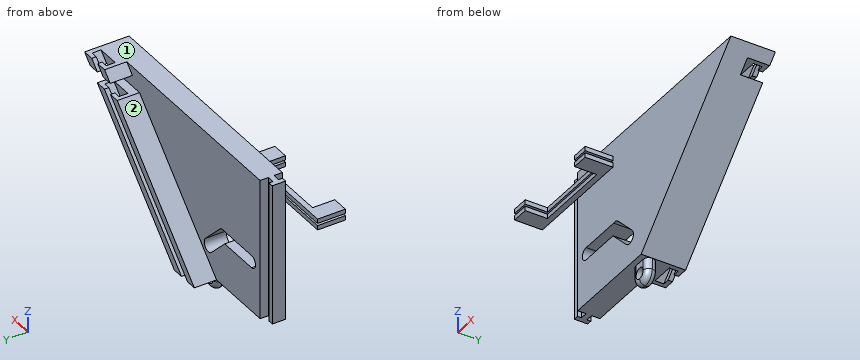
```python
from build123d import *

# Parameters (mm, degrees)
BOSS_EXTRUDE1_DEPTH  = 10
BOSS_EXTRUDE3_DEPTH  = 65
SKETCH3_W            = 6.566984135
SKETCH3_H            = 1.360389693
CUT_EXTRUDE2_DEPTH   = 65
BOSS_EXTRUDE4_DEPTH  = 3.25
BOSS_EXTRUDE5_DEPTH  = 2.25
SKETCH7_W            = 10
SKETCH7_H            = 5
BOSS_EXTRUDE6_DEPTH  = 10
SKETCH8_R            = 2.5
CUT_EXTRUDE3_DEPTH   = 10
FILLET1_R            = 5
FILLET2_R            = 5
FILLET4_R            = 2.5
FILLET5_R            = 2.5
SKETCH9_W            = 100
SKETCH9_H            = 5.5
CUT_EXTRUDE4_DEPTH   = 100
BOSS_EXTRUDE7_DEPTH  = 10
CUT_EXTRUDE5_DEPTH   = 150
SKETCH12_W           = 29.92089387
SKETCH12_H           = 33.203721342
CUT_EXTRUDE6_DEPTH   = 150
SKETCH14_W           = 19.184954217
SKETCH14_H           = 28.132637814
CUT_EXTRUDE7_DEPTH   = 150
SKETCH16_W           = 15.620456736
SKETCH16_H           = 10.822807293
CUT_EXTRUDE8_DEPTH   = 150
CUT_EXTRUDE9_DEPTH   = 10
CUT_EXTRUDE10_DEPTH  = 10
SKETCH19_W           = 10
SKETCH19_H           = 2
SKETCH19_W_2         = 15
BOSS_EXTRUDE9_DEPTH  = 2.5
SKETCH21_W           = 7.5
SKETCH21_H           = 2
BOSS_EXTRUDE10_DEPTH = 10


with BuildPart() as part:
    # Sketch1 → Boss-Extrude1 (new body)
    with BuildSketch(Plane(origin=(0, 0, 0), x_dir=(1, 0, 0), z_dir=(0, 1, 0))):
        Polygon((-11.672910159, -34.563988547), (96.966700148, -34.563988547), (33.327089841, 29.07562176), (-11.672910159, 29.07562176), align=None)
    extrude(amount=BOSS_EXTRUDE1_DEPTH)

    # Sketch2 → Boss-Extrude3 (add)
    with BuildSketch(Plane.XY.offset(34.563988547)):
        Polygon((-11.672910159, 3.75), (-14.922910159, 3.75), (-14.922910159, 2), (-17.172910159, 2), (-17.172910159, 8), (-14.922910159, 8), (-14.922910159, 6.25), (-11.672910159, 6.25), align=None)
    extrude(amount=-BOSS_EXTRUDE3_DEPTH)

    # Sketch3 → Cut-Extrude2 (cut)
    with BuildSketch(Plane(origin=(0, 8, 0), x_dir=(1, 0, 0), z_dir=(0, 1, 0))):
        with Locations((-13.889418092, 29.755816607)):
            Rectangle(SKETCH3_W, SKETCH3_H)
    extrude(amount=-CUT_EXTRUDE2_DEPTH, mode=Mode.SUBTRACT)

    # Sketch4 → Boss-Extrude4 (add)
    with BuildSketch(Plane(origin=(0, 10, 0), x_dir=(1, 0, 0), z_dir=(0, 1, 0))):
        Polygon((91.663399289, -34.563988547), (28.023788982, 29.07562176), (25.520630977, 29.07562176), (89.160241283, -34.563988547), align=None)
    extrude(amount=BOSS_EXTRUDE4_DEPTH)

    # Sketch6 → Boss-Extrude5 (add)
    with BuildSketch(Plane(origin=(0, 13.25, 0), x_dir=(1, 0, 0), z_dir=(0, 1, 0))):
        Polygon((90.411820286, -34.563988547), (94.136820286, -34.563988547), (30.497209979, 29.07562176), (23.047209979, 29.07562176), (86.686820286, -34.563988547), align=None)
    extrude(amount=BOSS_EXTRUDE5_DEPTH)

    # Sketch7 → Boss-Extrude6 (add)
    with BuildSketch(Plane(origin=(0, 0, -29.07562176), x_dir=(-1, 0, 0), z_dir=(0, 0, -1))):
        with Locations((-28.327089841, 5)):
            Rectangle(SKETCH7_W, SKETCH7_H)
    extrude(amount=BOSS_EXTRUDE6_DEPTH)

    # Sketch8 → Cut-Extrude3 (cut)
    with BuildSketch(Plane(origin=(0, 7.5, 0), x_dir=(1, 0, 0), z_dir=(0, 1, 0))):
        with Locations(Location((28.327089841, 34.07562176, 0), (0, 0, 270))):
            Circle(SKETCH8_R)
    extrude(amount=-CUT_EXTRUDE3_DEPTH, mode=Mode.SUBTRACT)

    # Fillet1
    fillet1_edges = [part.edges().sort_by_distance(p)[0] for p in [
        (23.327089841, 5, -39.07562176),
    ]]
    fillet(fillet1_edges, radius=FILLET1_R)

    # Fillet2
    fillet2_edges = [part.edges().sort_by_distance(p)[0] for p in [
        (33.327089841, 5, -39.07562176),
    ]]
    fillet(fillet2_edges, radius=FILLET2_R - 0.0001)  # a hair under: the kernel refuses the full size

    # Fillet4
    fillet4_edges = [part.edges().sort_by_distance(p)[0] for p in [
        (23.327089841, 7.5, -31.57562176),
        (33.327089841, 7.5, -31.57567176),
        (24.791555935, 7.5, -37.611155666),
    ]]
    fillet(fillet4_edges, radius=FILLET4_R - 0.0001)  # a hair under: the kernel refuses the full size

    # Fillet5
    fillet5_edges = [part.edges().sort_by_distance(p)[0] for p in [
        (23.327089841, 2.5, -31.57562176),
        (33.327089841, 2.5, -31.57567176),
        (24.791555935, 2.5, -37.611155666),
        (31.862653036, 2.5, -37.611184955),
    ]]
    fillet(fillet5_edges, radius=FILLET5_R - 0.0001)  # a hair under: the kernel refuses the full size

    # Sketch9 → Cut-Extrude4 (cut)
    with BuildSketch(Plane.XY.offset(34.563988547)):
        with Locations((44.136820286, 12.75)):
            Rectangle(SKETCH9_W, SKETCH9_H)
    extrude(amount=-CUT_EXTRUDE4_DEPTH, mode=Mode.SUBTRACT)

    # Sketch10 → Boss-Extrude7 (add)
    with BuildSketch(Plane(origin=(0, 10, 0), x_dir=(1, 0, 0), z_dir=(0, 1, 0))):
        Polygon((96.966700148, -34.563988547), (89.895632336, -41.635056358), (7.416994707, 40.84358127), (14.488062519, 47.914649082), align=None)
    extrude(amount=BOSS_EXTRUDE7_DEPTH)

    # Sketch11 → Cut-Extrude5 (cut)
    with BuildSketch(Plane(origin=(65.765344347, 0, 65.765344347), x_dir=(0.7071067811865475, 0, -0.7071067811865477), z_dir=(0.7071067811865477, 0, 0.7071067811865475))):
        Polygon((40.542543722, 20), (40.542543722, 18), (42.592543722, 18), (42.592543722, 14), (35.492543722, 14), (35.492543722, 18), (37.542543722, 18), (37.542543722, 20), align=None)
    extrude(amount=-CUT_EXTRUDE5_DEPTH, mode=Mode.SUBTRACT)

    # Sketch12 → Cut-Extrude6 (cut)
    with BuildSketch(Plane(origin=(0, 10, 0), x_dir=(-1, 0, 0), z_dir=(0, -1, 0))):
        with Locations((-34.145401152, 45.677482431)):
            Rectangle(SKETCH12_W, SKETCH12_H)
    extrude(amount=-CUT_EXTRUDE6_DEPTH, mode=Mode.SUBTRACT)


with BuildPart() as cut_extrude6_piece_1:
    # of the separate pieces the step leaves, piece 1, a body of its own (cut_extrude6_pieces)
    add(part.part.solids().sort_by_distance((30.827189841, 2.5, -29.07562176))[0])

    # Sketch16 → Cut-Extrude8 (cut)
    with BuildSketch(Plane(origin=(0, 10, 0), x_dir=(-1, 0, 0), z_dir=(0, -1, 0))):
        with Locations((-90.634792892, -39.975392193)):
            Rectangle(SKETCH16_W, SKETCH16_H)
    extrude(amount=-CUT_EXTRUDE8_DEPTH, mode=Mode.SUBTRACT)

    # Sketch17 → Cut-Extrude9 (cut)
    with BuildSketch(Plane(origin=(0, 20, 0), x_dir=(1, 0, 0), z_dir=(0, 1, 0))):
        Polygon((92.966700148, -30.563988547), (78.824564524, -30.563988547), (73.824564524, -25.563988547), (87.966700148, -25.563988547), align=None)
    extrude(amount=-CUT_EXTRUDE9_DEPTH, mode=Mode.SUBTRACT)

    # Sketch18 → Cut-Extrude10 (cut)
    with BuildSketch(Plane(origin=(0, 10, 0), x_dir=(1, 0, 0), z_dir=(0, 1, 0))):
        with BuildLine():
            Line((27.059004739, 14.493613639), (16.811162643, 4.245771544))
            ThreePointArc((16.811162643, 4.245771544), (12.674223335, 4.245771544), (12.674223335, 8.382710852))
            Line((12.674223335, 8.382710852), (22.92206543, 18.630552948))
            ThreePointArc((22.92206543, 18.630552948), (27.059004739, 18.630552948), (27.059004739, 14.493613639))
        make_face()
        with BuildLine():
            Line((14.742692989, 3.517272066), (-5.595455146, 3.517272066))
            ThreePointArc((-5.595455146, 3.517272066), (-8.392424278, 6.314241198), (-5.595455146, 9.11121033))
            Line((-5.595455146, 9.11121033), (14.742692989, 9.11121033))
            ThreePointArc((14.742692989, 9.11121033), (17.539662121, 6.314241198), (14.742692989, 3.517272066))
        make_face()
    extrude(amount=-CUT_EXTRUDE10_DEPTH, mode=Mode.SUBTRACT)

    # Sketch19 → Boss-Extrude9 (add)
    with BuildSketch(Plane(origin=(0, 0, 0), x_dir=(-1, 0, 0), z_dir=(0, -1, 0))):
        with Locations((-8.327089841, -26.563988547)):
            Rectangle(SKETCH19_W, SKETCH19_H)
        with Locations((-8.327089841, -23.563988547)):
            Rectangle(SKETCH19_W, SKETCH19_H)
        with Locations((31.672910159, -26.563988547)):
            Rectangle(SKETCH19_W, SKETCH19_H)
        with Locations((31.672910159, -23.563988547)):
            Rectangle(SKETCH19_W, SKETCH19_H)
        with Locations((4.172910159, -26.563988547)):
            Rectangle(SKETCH19_W_2, SKETCH19_H)
        with Locations((4.172910159, -23.563988547)):
            Rectangle(SKETCH19_W_2, SKETCH19_H)
        with Locations((19.172910159, -26.563988547)):
            Rectangle(SKETCH19_W_2, SKETCH19_H)
        with Locations((19.172910159, -23.563988547)):
            Rectangle(SKETCH19_W_2, SKETCH19_H)
    extrude(amount=BOSS_EXTRUDE9_DEPTH)

    # Sketch21 → Boss-Extrude10 (add)
    with BuildSketch(Plane(origin=(0, -2.5, 0), x_dir=(-1, 0, 0), z_dir=(0, -1, 0))):
        with Locations((-9.577089841, -23.563988547)):
            Rectangle(SKETCH21_W, SKETCH21_H)
        with Locations((-9.577089841, -26.563988547)):
            Rectangle(SKETCH21_W, SKETCH21_H)
        with Locations((32.922910159, -26.563988547)):
            Rectangle(SKETCH21_W, SKETCH21_H)
        with Locations((32.922910159, -23.563988547)):
            Rectangle(SKETCH21_W, SKETCH21_H)
    extrude(amount=BOSS_EXTRUDE10_DEPTH)


with BuildPart() as cut_extrude6_piece_2:
    # of the separate pieces the step leaves, piece 2, a body of its own (cut_extrude6_pieces)
    add(part.part.solids().sort_by_distance((7.416994707, 10, -40.84358127))[0])

    # Sketch14 → Cut-Extrude7 (cut)
    with BuildSketch(Plane(origin=(0, 10, 0), x_dir=(-1, 0, 0), z_dir=(0, -1, 0))):
        with Locations((-9.592477109, 43.141940667)):
            Rectangle(SKETCH14_W, SKETCH14_H)
    extrude(amount=-CUT_EXTRUDE7_DEPTH, mode=Mode.SUBTRACT)


solid = cut_extrude6_piece_1.part
```
CAD build for the part. Positions are in the model's coordinates, mm. Face numbers are marked on the shaded views. A direction names the side the tool comes from. Round coordinates to 2 decimals unless told otherwise and drop trailing zeros. Order: outer loops, then holes, each group sorted by start corner. A loop starts at its lowest first (then second) coordinate and runs counter-clockwise, first axis right, second up. Notation, with made-up numbers: (11.5, -5.75) -> (69.5, -5.75) arc R21 cw to (69.5, 22.25) -> close; hole circle Ø3 at (82.5, 71.5). An arc over 180 degrees is marked (long way). Write item = value, one per line.
(1) Flat gauge pins, fed straight in: P1, Ø0.6, axis at x = -17.5, z = 23.5, coming from the -Y side; P2, Ø1.9, axis at y = 2, z = -8.5, coming from the -X side; P3, Ø12, axis at x = -10, z = -31.5, coming from the +Y side. Where does each tip first touch, or does it go through?
Answers follow:
P1 = -2.5
P2 = -17.17
P3 = 10
(2) Cut at D-D (z = 2). Write the cut outline in (x, y).
Answers follow:
outline = (-17.17, 2) -> (-14.92, 2) -> (-14.92, 3.75) -> (-11.67, 3.75) -> (-11.67, 0) -> (64.4, 0) -> (64.4, 20) -> (59.34, 20) -> (59.34, 18) -> (62.23, 18) -> (62.23, 14) -> (52.19, 14) -> (52.19, 18) -> (55.09, 18) -> (55.09, 20) -> (50.26, 20) -> (50.26, 10) -> (-11.67, 10) -> (-11.67, 6.25) -> (-14.92, 6.25) -> (-14.92, 8) -> (-17.17, 8) -> close
(3) Cut at B-B (y = -5). Write the cut outline in (x, z).
Answers follow:
outline = (-36.67, 22.56) -> (-29.17, 22.56) -> (-29.17, 24.56) -> (-36.67, 24.56) -> close; (-36.67, 25.56) -> (-29.17, 25.56) -> (-29.17, 27.56) -> (-36.67, 27.56) -> close; (5.83, 22.56) -> (13.33, 22.56) -> (13.33, 24.56) -> (5.83, 24.56) -> close; (5.83, 25.56) -> (13.33, 25.56) -> (13.33, 27.56) -> (5.83, 27.56) -> close
(4) Cut at A-A (z = -11). Write the cut outline in (x, y).
Answers follow:
outline = (-17.17, 2) -> (-14.92, 2) -> (-14.92, 3.75) -> (-11.67, 3.75) -> (-11.67, 0) -> (15.29, 0) -> (15.29, 10) -> (-11.67, 10) -> (-11.67, 6.25) -> (-14.92, 6.25) -> (-14.92, 8) -> (-17.17, 8) -> close; (23.57, 0) -> (51.4, 0) -> (51.4, 20) -> (46.34, 20) -> (46.34, 18) -> (49.23, 18) -> (49.23, 14) -> (39.19, 14) -> (39.19, 18) -> (42.09, 18) -> (42.09, 20) -> (37.26, 20) -> (37.26, 10) -> (23.57, 10) -> close
(5) 3-axis set-ups, long thin cutter, end or side, ignore diameter. For the marked faces 1 and 2: which of +Z, -Z, +X, -X, +Y, -Y reach the whole face in a straight line?
Answers follow:
face_1 = +Z, +X, -X, +Y, -Y
face_2 = +Z, -X, +Y
(6) Cut at C-C (x = 49.5). Write the cut outline in (y, z).
Answers follow:
outline = (0, -12.9) -> (20, -12.9) -> (20, -7.84) -> (18, -7.84) -> (18, -10.73) -> (14, -10.73) -> (14, -0.69) -> (18, -0.69) -> (18, -3.59) -> (20, -3.59) -> (20, 1.24) -> (10, 1.24) -> (10, 34.56) -> (0, 34.56) -> close
(7) Drill centre lines: L1, parallel to Y at x = 37, z = -14.5; L2, parallel to Z at x = 3.5, y = 1.5; L3, parallel to X at y = -2, z = 24.5. Where is each one in solid material? Low to high.
Answers follow:
L1 = 0 to 14, 18 to 20
L2 = -29.08 to -9.11, -3.52 to 34.56
L3 = -36.67 to 13.33
